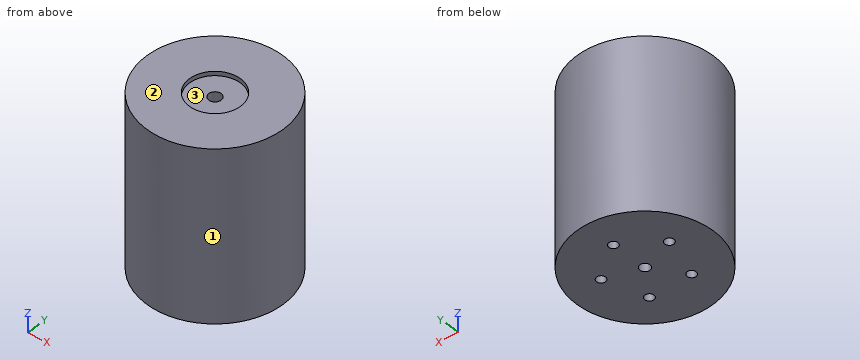
from build123d import *

# Parameters (mm, degrees)
F0_R     = 80
F1_DEPTH = 200
F3_D     = 14.5
F3_DEPTH = 40
F3_TIP   = 4.3562394879
F2_R     = 30
F2_R_2   = 20
F4_DEPTH = 5
F6_D     = 10.5
F6_DEPTH = 25
F6_TIP   = 3.1545182499
F7_D     = 12
F7_DEPTH = 25
F7_TIP   = 3.6051637142


with BuildPart() as f1:
    # F0 (on Top) → F1 (new body)
    with BuildSketch(Plane.XY):
        Circle(F0_R)
    extrude(amount=F1_DEPTH)

    # F3
    with Locations(Plane.XY.offset(200)):
        with Locations((0, 0)):
            Hole(F3_D / 2, depth=F3_DEPTH)
            with Locations((0, 0, -(F3_DEPTH + F3_TIP / 2))):  # 118° drill point
                Cone(0, F3_D / 2, F3_TIP, mode=Mode.SUBTRACT)

    # F2 (on face) → F4 (cut)
    with BuildSketch(Plane.XY.offset(200)):
        Circle(F2_R)
        Circle(F2_R_2, mode=Mode.SUBTRACT)
        Circle(F2_R_2)
    extrude(amount=-F4_DEPTH, mode=Mode.SUBTRACT)

    # F6
    with Locations(Plane(origin=(0, 0, 0), x_dir=(1, 0, 0), z_dir=(0, 0, -1))):
        with Locations((-24.9808732224, 34.3832222609), (-40.4199019425, -13.1332222609), (0, -42.5), (40.4199019425, -13.1332222609), (24.9808732224, 34.3832222609)):
            Hole(F6_D / 2, depth=F6_DEPTH)
            with Locations((0, 0, -(F6_DEPTH + F6_TIP / 2))):  # 118° drill point
                Cone(0, F6_D / 2, F6_TIP, mode=Mode.SUBTRACT)

    # F7
    with Locations(Plane(origin=(0, 0, 0), x_dir=(1, 0, 0), z_dir=(0, 0, -1))):
        with Locations((0, 0)):
            Hole(F7_D / 2, depth=F7_DEPTH)
            with Locations((0, 0, -(F7_DEPTH + F7_TIP / 2))):  # 118° drill point
                Cone(0, F7_D / 2, F7_TIP, mode=Mode.SUBTRACT)


solid = f1.part
Verification items for the finished model (mm, model axes). Face numbers are marked on the shaded views. Coordinates: 2 decimals unless noted, no trailing zeros. Write each loop counter-clockwise with the first axis right and the second up, starting at its lowest first coordinate (ties: lowest second). Pieces come first, ordered by that corner, then holes. Notation, with made-up numbers: (22, 2) -> (54, 2) arc R18 cw to (54, 28) -> close; hole circle Ø9 at (84, -39.5). An arc over 180 degrees is marked (long way). One line per item, written item: value. Start each with the question number.
Q1. Mould release check, pull along X, two halves, no side actions. Record for the marked faces 1, 2 and 3: pulls with the +X half, pulls with the -X half, needs draft (parallel to the pull), parting line crosses it, or undercut.
Q2. Thickness scan on L1, parallel to Y at x = 0, z = 6; L2, parallel to Y at x = 0, z = 179; L3, parallel to Z at x = -16.5, y = 12.5. Record the ranges inside material, lowest first. Write a range as from..to.
Q3. Cross-section at D-D on x = 61.5. Enter the section's corners in (y, z).
Q4. Cross-section at A-A on z = 34.5. Enter the section's corners in (x, y).
Q5. Cross-section at B-B on x = -15. Enter the section's corners in (y, z), and give its area (3 significant figures).
Q6. Go/stop test with flat-tipped pins: P1, Ø9.5, axis at x = -40.42, y = 13.13, coming from the -Z side; P2, Ø1, axis at x = -15.5, z = 45, coming from the -Y side; P3, Ø3, axis at x = 13.5, y = -10.5, coming from the +Z side. Record where each tip stops, or that it passes through.
Q7. Cross-section at C-C on y = -11. Enter the section's corners in (x, z), and give its area (3 significant figures).
Checked values:
1. face 1: parting line crosses it
1. face 2: needs draft
1. face 3: undercut
2. L1: y = -80..-6, 6..37.25, 47.75..80
2. L2: y = -80..-7.25, 7.25..80
2. L3: z = 0..195
3. outline: (-51.16, 0) -> (51.16, 0) -> (51.16, 200) -> (-51.16, 200) -> close
4. outline: circle Ø160 at (0, 0)
5. outline: (-78.58, 0) -> (78.58, 0) -> (78.58, 200) -> (25.98, 200) -> (25.98, 195) -> (-25.98, 195) -> (-25.98, 200) -> (-78.58, 200) -> close
5. area: 31,200 mm²
6. P1: stops at z = 25.3
6. P2: stops at y = -78.58
6. P3: stops at z = 195
7. outline: (-79.24, 0) -> (79.24, 0) -> (79.24, 200) -> (27.91, 200) -> (27.91, 195) -> (-27.91, 195) -> (-27.91, 200) -> (-79.24, 200) -> close
7. area: 31,400 mm²
